Model file for the job. Use its own axes, mm. A direction names the side the tool comes from. Give positions to 0.01 mm unless a question says otherwise; leave off trailing zeros. Loops run counter-clockwise (first coordinate to the right, second up) from the corner with the lowest first, then second, coordinate; pieces in that order, holes last. Notation, with made-up numbers: (-33, 80.25) - (-5, 80.25) arc R18 cw to (-5, 115.25) - close; hole circle Ø5 at (23.5, -34.75). An arc over 180 degrees is marked (long way). Use a Markdown table: item, result.
from build123d import *

# Parameters (mm, degrees)
SKETCH_1_W          = 72
SKETCH_1_H          = 12
EXTRUDE_1_DEPTH     = 3
CUT_EXTRUDE_1_DEPTH = 74.054773971
SKETCH_3_R          = 1.95
CUT_EXTRUDE_2_DEPTH = 74.054773971
FILLET_1_R          = 2


with BuildPart() as part:
    # 草图1 → 凸台-拉伸1 (new body)
    with BuildSketch(Plane.XY):
        with Locations((36, -6)):
            Rectangle(SKETCH_1_W, SKETCH_1_H)
    extrude(amount=EXTRUDE_1_DEPTH)

    # 草图2 → 切除-拉伸1 (cut, through all)
    with BuildSketch(Plane.XY.offset(3)):
        with BuildLine():
            Line((6, -4.5), (66, -4.5))
            ThreePointArc((66, -4.5), (67.5, -6), (66, -7.5))
            Line((66, -7.5), (6, -7.5))
            ThreePointArc((6, -7.5), (4.5, -6), (6, -4.5))
        make_face()
    extrude(amount=-CUT_EXTRUDE_1_DEPTH, mode=Mode.SUBTRACT)

    # 草图3 → 切除-拉伸2 (cut, through all)
    with BuildSketch(Plane.XY.offset(3)):
        with Locations((41, -6)):
            Circle(SKETCH_3_R)
        with Locations((31, -6)):
            Circle(SKETCH_3_R)
    extrude(amount=-CUT_EXTRUDE_2_DEPTH, mode=Mode.SUBTRACT)

    # 圆角1
    fillet_1_edges = [part.edges().sort_by_distance(p)[0] for p in [
        (0, 0, 1.5),
        (72, 0, 1.5),
        (72, -12, 1.5),
        (0, -12, 1.5),
    ]]
    fillet(fillet_1_edges, radius=FILLET_1_R)


solid = part.part
(1) Mould opens along Y. For faces 3 (the flat face through (35, -3, 0)), 4 (the cylindrical face through (0.57, -0.6, 1.52)), 5 (the flat face through (54, -4.5, 2)) say: pulls with the +Y half, pulls with the -Y half, needs draft (parallel to the pull), parting line crosses it, or undercut.
Computed:
| item | result |
|---|---|
| face 3 | needs draft |
| face 4 | pulls with the +Y half |
| face 5 | undercut |
(2) Slice it at C-C, the plane y = -6. Write the cut outline in (x, z).
Computed:
| item | result |
|---|---|
| outline | (0, 0) - (4.5, 0) - (4.5, 3) - (0, 3) - close; (67.5, 0) - (72, 0) - (72, 3) - (67.5, 3) - close |
(3) Slice it at A-A, the plane x = 51. Write the cut outline in (y, z).
Computed:
| item | result |
|---|---|
| outline | (-12, 0) - (-7.5, 0) - (-7.5, 3) - (-12, 3) - close; (-4.5, 0) - (0, 0) - (0, 3) - (-4.5, 3) - close |
(4) 3-axis set-ups, long thin cutter, end or side, ignore diameter. For faces 1 (the cylindrical face through (30.98, -7.95, 1.52)), 2 (the cylindrical face through (0.57, -11.4, 1.52)): which of +Z, -Z, +X, -X, +Y, -Y reach the whole face in a straight line?
Computed:
| item | result |
|---|---|
| face 1 | +Z, -Z |
| face 2 | +Z, -Z, -X, -Y |
(5) Slice it at B-B, the plane z = 0.45. Write the cut outline in (x, y).
Computed:
| item | result |
|---|---|
| outline | (0, -10) arc R2 ccw to (2, -12) - (70, -12) arc R2 ccw to (72, -10) - (72, -2) arc R2 ccw to (70, 0) - (2, 0) arc R2 ccw to (0, -2) - close; hole (6, -7.5) - (29.75, -7.5) arc R1.95 ccw to (32.25, -7.5) - (39.75, -7.5) arc R1.95 ccw to (42.25, -7.5) - (66, -7.5) arc R1.5 ccw to (66, -4.5) - (42.25, -4.5) arc R1.95 ccw to (39.75, -4.5) - (32.25, -4.5) arc R1.95 ccw to (29.75, -4.5) - (6, -4.5) arc R1.5 ccw to start |
(6) Drill centre lines: probe 1 along Y at (x, z) = (28, 1.7); probe 2 along X at (y, z) = (-6.75, 0.6); probe 3 along X at (y, z) = (-5.5, 2.85). Where is each one in solid material? Low to high. Write a range as [from, to].
Computed:
| item | result |
|---|---|
| probe 1 | [-12, -7.5], [-4.5, 0] |
| probe 2 | [0, 4.7], [67.3, 72] |
| probe 3 | [0, 4.59], [67.41, 72] |
